Check sheet for the modelled part. Datum: model origin and axes. Units: mm. A direction names the side the tool comes from. Coordinates: 2 decimals unless noted, no trailing zeros. Order: outer loops, then holes, each group sorted by start corner. A loop starts at its lowest first (then second) coordinate and runs counter-clockwise, first axis right, second up.
from build123d import *

# Parameters (mm, degrees)
SKETCH_2_R      = 1.6
EXTRUDE_1_DEPTH = 4


with BuildPart() as part:
    # ｽｹｯﾁ2 → ﾎﾞｽ - 押し出し1 (new body)
    with BuildSketch(Plane(origin=(0, 0, 0), x_dir=(1, 0, 0), z_dir=(0, 1, 0))):
        with BuildLine():
            Line((2.022542486, -1.469463131), (-3.267524785, -8.75061608))
            ThreePointArc((-3.267524785, -8.75061608), (-6.759530401, -9.303695435), (-7.312609757, -5.811689819))
            Line((-7.312609757, -5.811689819), (-6.850442022, -5.175570505))
            ThreePointArc((-6.850442022, -5.175570505), (-6.686462962, -3.092019001), (-8.468476011, -2))
            Line((-8.468476011, -2), (-19.061552813, -2))
            Line((-19.061552813, -2), (-19.061552813, 2))
            Line((-19.061552813, 2), (-2.061552813, 2))
            ThreePointArc((-2.061552813, 2), (-1.590148292, 2.056349368), (-1.145307118, 2.222222222))
            ThreePointArc((-1.145307118, 2.222222222), (1.897240274, 1.628029281), (2.022542486, -1.469463131))
        make_face()
        with Locations(Location((0, 0, 0), (0, 0, 270))):
            Circle(SKETCH_2_R, mode=Mode.SUBTRACT)
        with Locations(Location((-5.290067271, -7.281152949, 0), (0, 0, 270))):
            Circle(SKETCH_2_R, mode=Mode.SUBTRACT)
    extrude(amount=EXTRUDE_1_DEPTH)


solid = part.part
(1) Cross-section at C-C (y = 2.4). Enter the section's corners in (x, z), and give its area (3 significant figures).
Filled in:
outline: (-19.06, -2) - (-2.06, -2) arc R2 cw to (-1.15, -2.22) arc R2.5 ccw to (2.02, 1.47) - (-3.27, 8.75) arc R2.5 ccw to (-7.31, 5.81) - (-6.85, 5.18) arc R2 cw to (-8.47, 2) - (-19.06, 2) - close; hole circle Ø3.2 at (-5.29, 7.28); hole circle Ø3.2 at (0, 0)
area: 116 mm2
(2) Thickness scan on probe 1 along X at (y, z) = (1.35, 0); probe 2 along Z at (x, y) = (-17.25, 2.45); probe 3 along X at (y, z) = (1.1, 6.75). Record the ranges inside material, lowest first.
Filled in:
probe 1: x = -19.06 to -1.6, 1.6 to 2.5
probe 2: z = -2 to 2
probe 3: x = -7.73 to -6.8, -3.78 to -1.81
(3) Cross-section at B-B (x = 0). Enter the section's corners in (y, z), and give its area (3 significant figures).
Filled in:
outline: (0, -2.5) - (4, -2.5) - (4, -1.6) - (0, -1.6) - close; (0, 1.6) - (4, 1.6) - (4, 4.25) - (0, 4.25) - close
area: 14.2 mm2
(4) Cross-section at A-A (z = 0). Enter the section's corners in (x, y), and give its area (3 significant figures).
Filled in:
outline: (-19.06, 0) - (-1.6, 0) - (-1.6, 4) - (-19.06, 4) - close; (1.6, 0) - (2.5, 0) - (2.5, 4) - (1.6, 4) - close
area: 73.4 mm2
(5) Release check for a two-part mould opening along Z. For faces 1 (the cylindrical face through (-6.673, 1.972, 3.12)), 2 (the flat face through (-8, 0, 1)), 3 (the flat face through (-14, 2, 2)) record: +Z half, -Z half, draft (parallel to the pull), parting line (faces both ways), or undercut.
Filled in:
face 1: undercut
face 2: draft
face 3: +Z half
(6) Tool access check on faces 4 (the flat face through (-11, 2, -2)), 5 (the flat face through (-0.585, 1.972, 5.059)). Record the directions out of +Z, -Z, +X, -X, +Y, -Y that give a thin tool (end or side, any length) a straight path to the whole face; none if there is none.
Filled in:
face 4: -Z, -X, +Y, -Y
face 5: +Z, +X, +Y, -Y
(7) Go/stop test with flat-tipped pins: P1, Ø1.2, axis at x = -12.5, y = 2.5, coming from the +Z side; P2, Ø1, axis at x = -3, y = 2, coming from the -Z side. Record where each tip stops, or that it passes through.
Filled in:
P1: stops at z = 2
P2: stops at z = -2
